Can you work these out from the model? Positions are in its coordinate system, mm. Give positions to 0.01 mm unless a question says otherwise; leave off trailing zeros. Write each loop counter-clockwise with the first axis right and the second up, starting at its lowest first coordinate (ties: lowest second). Pieces come first, ordered by that corner, then holes.
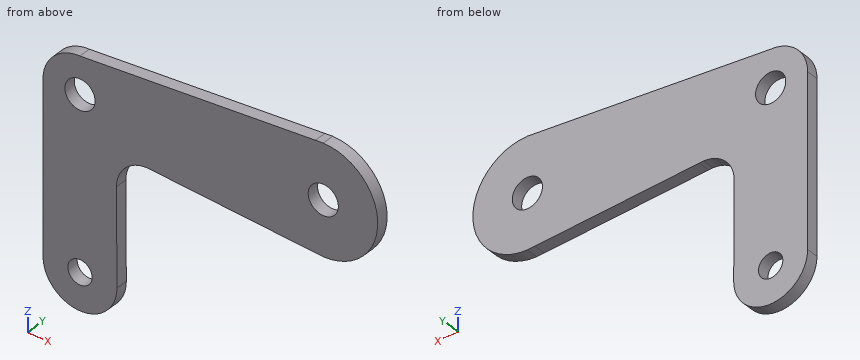
```python
from build123d import *

# Parameters (mm, degrees)
SKETCH1_R           = 3.937
SKETCH1_R_2         = 3.175
BOSS_EXTRUDE1_DEPTH = 3.175


with BuildPart() as part:
    # Sketch1 → Boss-Extrude1 (new body)
    with BuildSketch(Plane(origin=(0, 0, 0), x_dir=(1, 0, 0), z_dir=(0, 1, 0))):
        with BuildLine():
            ThreePointArc((-47.439743119, 21.70075638), (-57.091743119, 31.35275638), (-66.743743119, 21.70075638))
            Line((-66.743743119, 21.70075638), (-66.743743119, -22.74924362))
            ThreePointArc((-66.743743119, -22.74924362), (-63.916737771, -29.574238272), (-57.091743119, -32.40124362))
            Line((-57.091743119, -32.40124362), (4.370564279, -36.826529753))
            Line((4.370564279, -36.826529753), (6.408256881, -36.97324362))
            ThreePointArc((6.408256881, -36.97324362), (20.632256881, -22.74924362), (6.408256881, -8.52524362))
            Line((6.408256881, -8.52524362), (4.452941658, -8.660279201))
            Line((4.452941658, -8.660279201), (-38.465878307, -11.624286105))
            ThreePointArc((-38.465878307, -11.624286105), (-39.014500852, -11.681231653), (-39.565743119, -11.70024362))
            ThreePointArc((-39.565743119, -11.70024362), (-45.223304476, -9.356804976), (-47.566743119, -3.69924362))
            Line((-47.566743119, -3.69924362), (-47.566343079, -3.61923562))
            Line((-47.566343079, -3.61923562), (-47.440225707, 21.604238793))
            Line((-47.440225707, 21.604238793), (-47.439743119, 21.70075638))
        make_face()
        with Locations(Location((-57.091743119, -22.74924362, 0), (0, 0, 270))):
            Circle(SKETCH1_R, mode=Mode.SUBTRACT)
        with Locations(Location((6.408256881, -22.74924362, 0), (0, 0, 270))):
            Circle(SKETCH1_R, mode=Mode.SUBTRACT)
        with Locations(Location((-57.091743119, 21.70075638, 0), (0, 0, 270))):
            Circle(SKETCH1_R_2, mode=Mode.SUBTRACT)
    extrude(amount=-BOSS_EXTRUDE1_DEPTH)


solid = part.part
```
1) Suppose I cut it at A-A on z = 24. Write out the boundary of the cut face in (x, y) (3 decimals), plus the area to 3 significant figures.
Values follow:
outline: (-66.662, -3.175) - (-60.825, -3.175) - (-60.825, 0) - (-66.662, 0) - close; (-53.359, -3.175) - (2.675, -3.175) - (2.675, 0) - (-53.359, 0) - close; (10.141, -3.175) - (20.577, -3.175) - (20.577, 0) - (10.141, 0) - close
area: 230 mm2
2) Suppose I cut it at B-B on y = -2.25. Write out the boundary of the cut face in (x, z) (3 decimals), plus the area to 3 significant figures.
Values follow:
outline: (-66.744, -21.701) arc R9.652 ccw to (-47.44, -21.701) - (-47.567, 3.699) arc R8.001 cw to (-38.466, 11.624) - (6.408, 8.525) arc R14.224 ccw to (6.408, 36.973) - (-57.092, 32.401) arc R9.652 ccw to (-66.744, 22.749) - close; hole circle Ø7.874 at (-57.092, 22.749); hole circle Ø6.35 at (-57.092, -21.701); hole circle Ø7.874 at (6.408, 22.749)
area: 2,700 mm2
3) Please list where these lines run through material, in increasing order: L1, parallel to Z at x = -57.5, y = -0.15; L2, parallel to Z at x = -60, y = -3; L3, parallel to X at y = -1.5, z = -17.5.
Values follow:
L1: z = -31.34 to -24.85, -18.55 to 18.83, 26.67 to 32.39
L2: z = -30.9 to -22.97, -20.43 to 20.1, 25.4 to 31.95
L3: x = -66.74 to -47.46
4) For pin 1 Ø4 at (x, z) = (-48, 20) entering from +Y, with a flat end and sliding along its axis, tell me the tip position at first contact or that it passes through.
Values follow:
pin 1: stops at y = 0
5) Suppose I cut it at D-D on z = 16.5. Write out the boundary of the cut face in (x, y) (3 decimals), plus the area to 3 significant figures.
Values follow:
outline: (-66.744, -3.175) - (19.186, -3.175) - (19.186, 0) - (-66.744, 0) - close
area: 273 mm2
6) Suppose I cut it at C-C on x = -58. Write out the boundary of the cut face in (y, z) (3 decimals), plus the area to 3 significant figures.
Values follow:
outline: (-3.175, -31.31) - (0, -31.31) - (0, -24.743) - (-3.175, -24.743) - close; (-3.175, -18.658) - (0, -18.658) - (0, 18.918) - (-3.175, 18.918) - close; (-3.175, 26.58) - (0, 26.58) - (0, 32.358) - (-3.175, 32.358) - close
area: 159 mm2
